```python
from build123d import *

# Parameters (mm, degrees)
SKETCH1_R           = 3.25
BOSS_EXTRUDE1_DEPTH = 7.018
SKETCH6_R           = 4.7
BOSS_EXTRUDE2_DEPTH = 10
FILLET1_R           = 0.75
BOSS_EXTRUDE3_DEPTH = 1
BOSS_EXTRUDE4_DEPTH = 2


with BuildPart() as part:
    # Sketch1 → Boss-Extrude1 (new body)
    with BuildSketch(Plane(origin=(0, 0, 0), x_dir=(1, 0, 0), z_dir=(0, 1, 0))):
        Circle(SKETCH1_R)
    extrude(amount=BOSS_EXTRUDE1_DEPTH)

    # Sketch6 → Boss-Extrude2 (add)
    with BuildSketch(Plane(origin=(0, 7.018, 0), x_dir=(1, 0, 0), z_dir=(0, 1, 0))):
        Circle(SKETCH6_R)
    extrude(amount=BOSS_EXTRUDE2_DEPTH)

    # Fillet1
    fillet1_edges = [part.edges().sort_by_distance(p)[0] for p in [
        (-4.7, 17.018, 0),
    ]]
    fillet(fillet1_edges, radius=FILLET1_R)

    # Sketch8 → Boss-Extrude3 (add)
    with BuildSketch(Plane(origin=(0, 17.018, 0), x_dir=(1, 0, 0), z_dir=(0, 1, 0))):
        Polygon((0, 0.75), (-3, 0.75), (-3, -0.75), (0, -0.75), (0, -1.732050808), (3, 0), (0, 1.732050808), align=None)
    extrude(amount=BOSS_EXTRUDE3_DEPTH)

    # Sketch9 → Boss-Extrude4 (add)
    with BuildSketch(Plane.XZ.offset(-7.018)):
        with BuildLine():
            Line((-1.016, 4.588871757), (-1.016, 6.620871757))
            Line((-1.016, 6.620871757), (1.016, 6.620871757))
            Line((1.016, 6.620871757), (1.016, 4.588871757))
            ThreePointArc((1.016, 4.588871757), (0, 4.7), (-1.016, 4.588871757))
        make_face()
        with BuildLine():
            Line((-1.651, -4.400477133), (-1.651, -6.432477133))
            Line((-1.651, -6.432477133), (1.651, -6.432477133))
            Line((1.651, -6.432477133), (1.651, -4.400477133))
            ThreePointArc((1.651, -4.400477133), (0, -4.7), (-1.651, -4.400477133))
        make_face()
    extrude(amount=-BOSS_EXTRUDE4_DEPTH)


solid = part.part
```
Part model, mm, in its own coordinate system. A direction names the side the tool comes from. Round coordinates to 2 decimals unless told otherwise and drop trailing zeros. Loops run counter-clockwise (first coordinate to the right, second up) from the corner with the lowest first, then second, coordinate; pieces in that order, holes last.
Item 1: Drill centre lines: line 1 (Y direction, x = 1.75, z = -3.5); line 2 (Z direction, x = -2.75, y = 4.75); line 3 (Y direction, x = 0, z = 2.25). Where is each one in solid material? Low to high.
Item 2: 3-axis set-ups, long thin cutter, end or side, ignore diameter. For faces 1 (the face through (1.479, 17.511, 0.878)), 2 (the face through (-3, 7.018, -2)), 3 (the face through (1.651, 8, -5)), 4 (the face through (-3, 17.5, 0)), 5 (the face through (-1.5, 17.5, 0.75)): which of +Z, -Z, +X, -X, +Y, -Y reach the whole face in a straight line?
Item 3: Drop flat-ended pins along their axis: P1, Ø1, axis at x = 0.5, z = 5, coming from the +Y side; P2, Ø2, axis at y = 7.5, z = -5.5, coming from the +X side; P3, Ø1.5, axis at x = -1.5, y = 4, coming from the -Z side; P4, Ø4, axis at x = 0.5, z = 1.5, coming from the +Y side. Give the stop position or say it passes through.
Item 4: Cut at B-B, the plane z = -5.25. Give the cut face in (x, y), then the cut area to 3 significant figures.
Item 5: Cut at D-D, the plane y = 1.5. Give the cut face in (x, z).
Item 6: Cut at A-A, the plane y = 8. Give the cut face in (x, z), then the cut area to 3 significant figures.
Item 7: Cut at C-C, the plane y = 11. Give the cut face in (x, z).
A:
1. line 1: y = 7.02 to 17.02
1. line 2: z = -1.73 to 1.73
1. line 3: y = 0 to 17.02
2. face 1: +Z, +X, +Y
2. face 2: -Y
2. face 3: -Z, +X, +Y, -Y
2. face 4: +Z, -Z, -X, +Y
2. face 5: +Z, -X, +Y
3. P1: stops at y = 16.75
3. P2: stops at x = 1.65
3. P3: stops at z = -3.16
3. P4: stops at y = 18.02
4. outline: (-1.65, 7.02) - (1.65, 7.02) - (1.65, 9.02) - (-1.65, 9.02) - close
4. area: 6.60 mm2
5. outline: circle Ø6.5 at (0, 0)
6. outline: (-1.65, -6.43) - (1.65, -6.43) - (1.65, -4.4) arc R4.7 ccw to (1.02, 4.59) - (1.02, 6.62) - (-1.02, 6.62) - (-1.02, 4.59) arc R4.7 ccw to (-1.65, -4.4) - close
6. area: 79.4 mm2
7. outline: circle Ø9.4 at (0, 0)
